Verification items for the finished model (mm, model axes). A direction names the side the tool comes from. Round coordinates to 2 decimals unless told otherwise and drop trailing zeros. Order: outer loops, then holes, each group sorted by start corner. A loop starts at its lowest first (then second) coordinate and runs counter-clockwise, first axis right, second up. Notation, with made-up numbers: M -1.75,-2.5 L 46.25,-2.5 A22 ccw 46.25,33.5 Z; hole C -15.5,33.5 d8. An arc over 180 degrees is marked long. Answer as a JSON object with one key per item and string values. Group by question number.
```python
from build123d import *

# Parameters (mm, degrees)
ESQUISSE1_R        = 1.75
BOSS_EXTRU_1_DEPTH = 1.72
CONG_1_R           = 4
ESQUISSE2_W        = 165
ESQUISSE2_H        = 100
BOSS_EXTRU_2_DEPTH = 6.79
ESQUISSE3_W        = 12.17
ESQUISSE3_H        = 15.1
BOSS_EXTRU_3_DEPTH = 6.19
ESQUISSE4_W        = 5.85
ESQUISSE4_H        = 7.52
BOSS_EXTRU_4_DEPTH = 2.55
BOSS_EXTRU_5_START = 8
ESQUISSE5_R        = 1.75
BOSS_EXTRU_5_DEPTH = 8


with BuildPart() as part:
    # Esquisse1 → Boss.-Extru.1 (new body)
    with BuildSketch(Plane.XY):
        Polygon((-74.5, 53.5), (74.5, 53.5), (74.5, 62), (82.5, 62), (82.5, -62), (74.5, -62), (74.5, -53.5), (-74.5, -53.5), (-74.5, -62), (-82.5, -62), (-82.5, 62), (-74.5, 62), align=None)
        with Locations((78.5, 57.54)):
            Circle(ESQUISSE1_R, mode=Mode.SUBTRACT)
        with Locations((-78.4, 57.54)):
            Circle(ESQUISSE1_R, mode=Mode.SUBTRACT)
        with Locations((-78.4, -57.54)):
            Circle(ESQUISSE1_R, mode=Mode.SUBTRACT)
        with Locations((78.5, -57.54)):
            Circle(ESQUISSE1_R, mode=Mode.SUBTRACT)
    extrude(amount=BOSS_EXTRU_1_DEPTH)

    # Congé1
    cong_1_edges = [part.edges().sort_by_distance(p)[0] for p in [
        (74.5, -62, 0.86),
        (82.5, -62, 0.86),
        (82.5, 62, 0.86),
        (74.5, 62, 0.86),
        (-74.5, 62, 0.86),
        (-82.5, 62, 0.86),
        (-82.5, -62, 0.86),
        (-74.5, -62, 0.86),
    ]]
    fillet(cong_1_edges, radius=CONG_1_R - 0.0001)  # a hair under: the kernel refuses the full size

    # Esquisse2 → Boss.-Extru.2 (add)
    with BuildSketch(Plane.XY.offset(1.72)):
        with Locations((0, 3.1)):
            Rectangle(ESQUISSE2_W, ESQUISSE2_H)
    extrude(amount=BOSS_EXTRU_2_DEPTH)

    # Esquisse3 → Boss.-Extru.3 (add)
    with BuildSketch(Plane(origin=(0, 0, 0), x_dir=(-1, 0, 0), z_dir=(0, 0, -1))):
        with Locations((-77.485, 40.95)):
            Rectangle(ESQUISSE3_W, ESQUISSE3_H)
    extrude(amount=BOSS_EXTRU_3_DEPTH)

    # Esquisse4 → Boss.-Extru.4 (add)
    with BuildSketch(Plane(origin=(0, 0, 0), x_dir=(-1, 0, 0), z_dir=(0, 0, -1))):
        with Locations((-80.825, 22.14)):
            Rectangle(ESQUISSE4_W, ESQUISSE4_H)
        with Locations((-80.825, 7.12)):
            Rectangle(ESQUISSE4_W, ESQUISSE4_H)
    extrude(amount=BOSS_EXTRU_4_DEPTH)

    # Esquisse5 → Boss.-Extru.5 (add)
    # profile 1 of 4: a face of its own
    with BuildSketch(Plane(origin=(0, 0, 0), x_dir=(-1, 0, 0), z_dir=(0, 0, -1)).offset(BOSS_EXTRU_5_START)):
        Polygon((-78.5, -54.826453735), (-80.85, -56.183226867), (-80.85, -58.896773133), (-78.5, -60.253546265), (-76.15, -58.896773133), (-76.15, -56.183226867), align=None)
        with Locations((-78.5, -57.54)):
            Circle(ESQUISSE5_R, mode=Mode.SUBTRACT)
    # profile 2 of 4: a face of its own
    with BuildSketch(Plane(origin=(0, 0, 0), x_dir=(-1, 0, 0), z_dir=(0, 0, -1)).offset(BOSS_EXTRU_5_START)):
        Polygon((-78.5, 60.253546265), (-80.85, 58.896773133), (-80.85, 56.183226867), (-78.5, 54.826453735), (-76.15, 56.183226867), (-76.15, 58.896773133), align=None)
        with Locations((-78.5, 57.54)):
            Circle(ESQUISSE5_R, mode=Mode.SUBTRACT)
    # profile 3 of 4: a face of its own
    with BuildSketch(Plane(origin=(0, 0, 0), x_dir=(-1, 0, 0), z_dir=(0, 0, -1)).offset(BOSS_EXTRU_5_START)):
        Polygon((78.460826557, 60.252864439), (76.081003757, 58.949109563), (76.020177201, 56.236245124), (78.339173443, 54.827135561), (80.718996243, 56.130890437), (80.779822799, 58.843754876), align=None)
        with Locations((78.4, 57.54)):
            Circle(ESQUISSE5_R, mode=Mode.SUBTRACT)
    # profile 4 of 4: a face of its own
    with BuildSketch(Plane(origin=(0, 0, 0), x_dir=(-1, 0, 0), z_dir=(0, 0, -1)).offset(BOSS_EXTRU_5_START)):
        Polygon((78.4, -54.826453735), (76.05, -56.183226867), (76.05, -58.896773133), (78.4, -60.253546265), (80.75, -58.896773133), (80.75, -56.183226867), align=None)
        with Locations((78.4, -57.54)):
            Circle(ESQUISSE5_R, mode=Mode.SUBTRACT)
    extrude(amount=-BOSS_EXTRU_5_DEPTH)


solid = part.part
```
Q1. Cross-section at B-B, the plane y = 40. Record the cut outline in (x, z), then the cut area to 3 significant figures.
Q2. Cross-section at C-C, the plane z = 6.75. Record the cut outline in (x, y), then the cut area to 3 significant figures.
Q3. Release check for a two-part mould opening along Y. For faces 4 (the face through (78, 33.4, -3)), 5 (the face through (82.5, 1, 4)), 6 (the face through (81.359, -60.797, 0.872)) record: released by +Y, released by -Y, zero draft, split by the parting line, or undercut.
Q4. Cross-section at A-A, the plane x = 32. Record the cut outline in (y, z).
Q5. Tool access check on faces 1 (the face through (81, 22, -2.55)), 2 (the face through (-75.641, 60.797, 0.872)), 3 (the face through (-75.703, -60.859, 0.872)). Record the directions out of +Z, -Z, +X, -X, +Y, -Y that give a thin tool (end or side, any length) a straight path to the whole face; none if there is none.
Q6. Gauge pin test, flat ends, axial feed: pin 1 Ø4.5 at (x, y) = (81, 6.5) entering from -Z; pin 2 Ø3 at (y, z) = (45.5, -3) entering from +X; pin 3 Ø0.5 at (y, z) = (56.5, 1) entering from +X; pin 4 Ø3 at (x, y) = (78.5, 57.54) entering from -Z. Record the tip position at first contact, or that the pin passes through.
Q7. Cross-section at D-D, the plane y = 1. Record the cut outline in (x, z), then the cut area to 3 significant figures.
Q8. Thickness scan on line 1 (X direction, y = 57.54, z = -1.75); line 2 (Y direction, x = -78.4, z = -2.75); line 3 (Y direction, x = 78.5, z = 1.1). Record the ranges inside material, lowest first. Write a range as from..to.
Conclusion:
{
 "1": {"outline": "M -82.5,0 L 71.4,0 L 71.4,-6.19 L 83.57,-6.19 L 83.57,0 L 82.5,0 L 82.5,8.51 L -82.5,8.51 Z", "area": "1,480 mm2"},
 "2": {"outline": "M -82.5,-46.9 L 82.5,-46.9 L 82.5,53.1 L -82.5,53.1 Z", "area": "16,500 mm2"},
 "3": {"face 4": "undercut", "face 5": "zero draft", "face 6": "released by -Y"},
 "4": {"outline": "M -53.5,0 L 53.5,0 L 53.5,1.72 L 53.1,1.72 L 53.1,8.51 L -46.9,8.51 L -46.9,1.72 L -53.5,1.72 Z"},
 "5": {"face 1": "-Z, +X, -X", "face 2": "+Z, -Z, +Y", "face 3": "+Z, -Z, -Y"},
 "6": {"pin 1": "z = -2.55", "pin 2": "x = 83.57", "pin 3": "x = 82.5", "pin 4": "through"},
 "7": {"outline": "M -82.5,0 L 82.5,0 L 82.5,8.51 L -82.5,8.51 Z", "area": "1,400 mm2"},
 "8": {"line 1": "-80.75..-80.15, -76.65..-76.05, 76.15..76.75, 80.25..80.85", "line 2": "-60.25..-59.29, -55.79..-54.83, 54.86..55.79, 59.29..60.22", "line 3": "-62..-59.29, -55.79..55.79, 59.29..62"}
}
